Build history of the part. All positions in model axes, mm. Face numbers are marked on the shaded views. A direction names the side the tool comes from. Give positions to 0.01 mm unless a question says otherwise; leave off trailing zeros. Order: outer loops, then holes, each group sorted by start corner. A loop starts at its lowest first (then second) coordinate and runs counter-clockwise, first axis right, second up. Notation, with made-up numbers: M 78,84.25 L 89,84.25 A34 ccw 89,117.25 Z; hole C 86,22.5 d1. An arc over 180 degrees is marked long. Use CSV: the item, a comma, the result in double quotes. Start each with the question number.
Item 1: Pin check, flat tips, straight feed: P1, Ø1.4, axis at x = -1, y = 0.5, coming from the -Z side; P2, Ø3, axis at y = 6, z = 1.5, coming from the +X side; P3, Ø1.5, axis at x = 0.5, y = 5.5, coming from the +Z side. Stop position of each tip, or through.
Item 2: Two-plate mould, pull along Z, no slides. Class the marked faces 4, 5 and 6: pulls with the +Z half, pulls with the -Z half, needs draft (parallel to the pull), parting line crosses it, or undercut.
Item 3: Band-saw the part on B-B on z = 0. Write the cut outline in (x, y).
Item 4: Wall check: line 1 along Y through (x, z) = (-1.8, 1.85); line 2 along Y through (x, z) = (1.5, -0.8); line 3 along Z through (x, y) = (0.3, 1.25). Give the ranges that are in metal, low to high.
Item 5: Band-saw the part on C-C on x = 0. Write the cut outline in (y, z), plus the area to 3 significant figures.
Item 6: Band-saw the part on D-D on y = 3.75. Write the cut outline in (x, z), plus the area to 3 significant figures.
Item 7: Which spindle directions (+Z, -Z, +X, -X, +Y, -Y) get a long thin tool onto all of the face, cutting with end or side? Do the marked faces 1, 2 and 3. Say none if no direction does.
Item 8: Band-saw the part on A-A on y = 1. Write the cut outline in (x, z), plus the area to 3 significant figures.
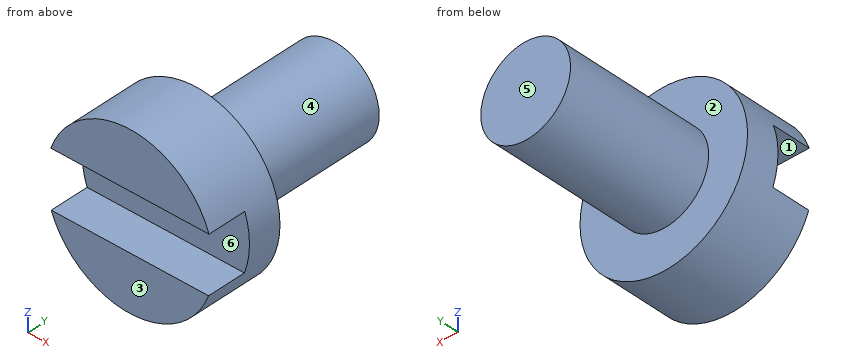
Autodesk Inventor part; units mm, degrees
ref_plane "YZ Plane" through (0, 0, 0) normal (1, 0, 0) x (0, 1, 0)
ref_plane "XZ Plane" through (0, 0, 0) normal (0, 1, 0) x (-1, 0, 0)
ref_plane "XY Plane" through (0, 0, 0) normal (0, 0, 1) x (1, 0, 0)
sketch "Esboço1" plane through (0, 0, 0) normal (0, 1, 0) x (-1, 0, 0)
  circle A0 centre (0, 0) radius 2.8
  dimension "d0" = 5.6
extrude "Extrusão1" add sketch "Esboço1" along normal blind 2.4
sketch "Esboço2" plane through (0, 0, 0) normal (1, 0, 0) x (0, 1, 0)
  line L0 (0, 0.9185) -> (1.2961, 0.9185)
  line L1 (1.2961, 0.9185) -> (1.2961, -0.9611)
  line L2 (1.2961, -0.9611) -> (0, -0.9611)
  line L3 (0, -0.9611) -> (0, 0.9185)
  point P0 (0, 0)
extrude "Extrusão2" cut sketch "Esboço2" along normal through all both and the other way through all
sketch "Esboço3" plane through (0, 2.4, 0) normal (0, 1, 0) x (1, 0, 0)
  circle A0 centre (0, 0) radius 2.8
  circle A1 centre (0, 0) radius 1.5
  dimension "d5" = 3
extrude "Extrusão3" add sketch "Esboço3" along normal blind 5 contours A1
thread "Rosca1"
properties part number "Parafuso-M3-5"
Model answer:
1,P1,"stops at z = -2.78"
1,P2,"stops at x = 1.5"
1,P3,"stops at z = 1.5"
2,face 4,"parting line crosses it"
2,face 5,"needs draft"
2,face 6,"undercut"
3,outline,"M -2.8,1.3 L 2.8,1.3 L 2.8,2.4 L 1.5,2.4 L 1.5,7.4 L -1.5,7.4 L -1.5,2.4 L -2.8,2.4 Z"
4,line 1,"y = 0 to 2.4"
4,line 2,"y = 1.3 to 2.4"
4,line 3,"z = -2.78 to -0.96, 0.92 to 2.78"
5,outline,"M 0,-2.8 L 2.4,-2.8 L 2.4,-1.5 L 7.4,-1.5 L 7.4,1.5 L 2.4,1.5 L 2.4,2.8 L 0,2.8 L 0,0.92 L 1.3,0.92 L 1.3,-0.96 L 0,-0.96 Z"
5,area,"26.0 mm^2"
6,outline,"C 0,0 d3"
6,area,"7.07 mm^2"
7,face 1,"+X, -X, -Y"
7,face 2,"+Y"
7,face 3,"+Z, -Z, +X, -X, -Y"
8,outline,"M -2.65,0.92 L 2.65,0.92 A2.8 ccw Z; M -2.63,-0.96 A2.8 ccw 2.63,-0.96 Z"
8,area,"14.3 mm^2"
